Could you check a few things on this model? Use its own coordinates, in mm. Face numbers are marked on the shaded views. Round coordinates to 2 decimals unless told otherwise and drop trailing zeros. Loops run counter-clockwise (first coordinate to the right, second up) from the corner with the lowest first, then second, coordinate; pieces in that order, holes last. Notation, with made-up numbers: (-24.75, 22.5) -> (34.25, 22.5) arc R35 cw to (34.25, 55.5) -> close; hole circle Ø4 at (27, -25.75). An arc over 180 degrees is marked (long way). Put each result on its own line as item: value. Start each with the question number.
1. Imagine slicing it at B-B, the plane y = -9. Please give me the cut outline in (x, z), and give its area (3 significant figures).
2. Imagine slicing it at D-D, the plane y = -12. Please give me the cut outline in (x, z).
3. If we mould it in two halves opening along X, with no side actions, what happens to the marked faces 1, 2 and 3? For each: pulls with the +X half, pulls with the -X half, needs draft (parallel to the pull), parting line crosses it, or undercut.
4. Imagine slicing it at A-A, the plane z = 3.3. Please give me the cut outline in (x, y).
5. I'm going to push flat-ended pins straight in: P1, Ø1, axis at y = -19, z = 1, coming from the +X side; P2, Ø1, axis at y = -6.5, z = 1, coming from the -X side; P3, Ø0.6, axis at x = 0.5, y = -8.5, coming from the -Z side; P4, Ø2, axis at x = 7, z = 4, coming from the +Y side. Where does each tip first touch, or does it pass through?
6. Imagine slicing it at C-C, the plane x = 9. Please give me the cut outline in (y, z).
7. I need wall thicknesses on line 1 (Z direction, x = 28.5, y = -3); line 2 (X direction, y = -3.5, z = 1.4); line 3 (X direction, y = -10.5, z = 2.1). Which ranges of each line are inside material? Lowest first, please. Write a range as [from, to].
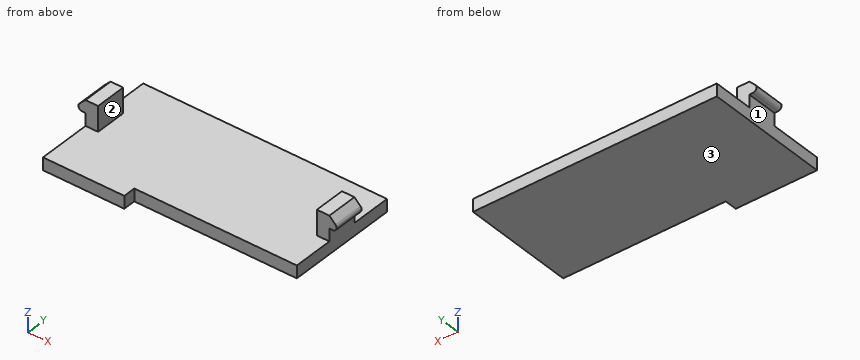
```python
from build123d import *

# Parameters (mm, degrees)
SKETCH1_W           = 40
SKETCH1_H           = 18
BOSS_EXTRUDE1_DEPTH = 2
SKETCH2_W           = 2
SKETCH2_H           = 5
BOSS_EXTRUDE2_DEPTH = 2
BOSS_EXTRUDE3_DEPTH = 5
FILLET1_R           = 0.6
SKETCH4_W           = 13
SKETCH4_H           = 2
BOSS_EXTRUDE4_DEPTH = 2
SKETCH5_W           = 1
SKETCH5_H           = 20
CUT_EXTRUDE1_DEPTH  = 10
SKETCH6_W           = 1
SKETCH6_H           = 2
BOSS_EXTRUDE5_DEPTH = 2


with BuildPart() as part:
    # Sketch1 → Boss-Extrude1 (new body)
    with BuildSketch(Plane.XY):
        with Locations((20, -9)):
            Rectangle(SKETCH1_W, SKETCH1_H)
    extrude(amount=BOSS_EXTRUDE1_DEPTH)

    # Sketch2 → Boss-Extrude2 (add)
    with BuildSketch(Plane.XY.offset(2)):
        with Locations((2, -9)):
            Rectangle(SKETCH2_W, SKETCH2_H)
        with Locations((39, -9)):
            Rectangle(SKETCH2_W, SKETCH2_H)
    extrude(amount=BOSS_EXTRUDE2_DEPTH)

    # Sketch3 → Boss-Extrude3 (add)
    with BuildSketch(Plane.XZ.offset(11.5)):
        Polygon((0, 4), (-1, 4), (1, 6), (3, 6), (3, 4), align=None)
        Polygon((38, 4), (38, 6), (40, 6), (42, 4), (40, 4), align=None)
    extrude(amount=-BOSS_EXTRUDE3_DEPTH)

    # Fillet1
    fillet1_edges = [part.edges().sort_by_distance(p)[0] for p in [
        (-1, -9, 4),
        (42, -9, 4),
    ]]
    fillet(fillet1_edges, radius=FILLET1_R)

    # Sketch4 → Boss-Extrude4 (add)
    with BuildSketch(Plane(origin=(0, 0, 0), x_dir=(-1, 0, 0), z_dir=(0, 0, -1))):
        with Locations((-6.5, -19)):
            Rectangle(SKETCH4_W, SKETCH4_H)
    extrude(amount=-BOSS_EXTRUDE4_DEPTH)

    # Sketch5 → Cut-Extrude1 (cut)
    with BuildSketch(Plane.XY.offset(2)):
        with Locations((0.5, -10)):
            Rectangle(SKETCH5_W, SKETCH5_H)
    extrude(amount=-CUT_EXTRUDE1_DEPTH, mode=Mode.SUBTRACT)

    # Sketch6 → Boss-Extrude5 (add)
    with BuildSketch(Plane.XY.offset(2)):
        with Locations((13.5, -19)):
            Rectangle(SKETCH6_W, SKETCH6_H)
    extrude(amount=-BOSS_EXTRUDE5_DEPTH)


solid = part.part
```
Entries:
1. outline: (0.02, 5.02) arc R0.6 ccw to (0.45, 4) -> (1, 4) -> (1, 0) -> (40, 0) -> (40, 4) -> (40.55, 4) arc R0.6 ccw to (40.98, 5.02) -> (40, 6) -> (38, 6) -> (38, 2) -> (3, 2) -> (3, 6) -> (1, 6) -> close
1. area: 97.1 mm^2
2. outline: (1, 0) -> (40, 0) -> (40, 2) -> (1, 2) -> close
3. face 1: pulls with the -X half
3. face 2: undercut
3. face 3: needs draft
4. outline: (1, -11.5) -> (3, -11.5) -> (3, -6.5) -> (1, -6.5) -> close; (38, -11.5) -> (40, -11.5) -> (40, -6.5) -> (38, -6.5) -> close
5. P1: x = 14
5. P2: x = 1
5. P3: z = 4
5. P4: through
6. outline: (-20, 0) -> (0, 0) -> (0, 2) -> (-20, 2) -> close
7. line 1: [0, 2]
7. line 2: [1, 40]
7. line 3: [1, 3], [38, 40]
